Autodesk Inventor part; units mm, degrees
ref_plane "YZ Plane" through (0, 0, 0) normal (1, 0, 0) x (0, 1, 0)
ref_plane "XZ Plane" through (0, 0, 0) normal (0, 1, 0) x (-1, 0, 0)
ref_plane "XY Plane" through (0, 0, 0) normal (0, 0, 1) x (1, 0, 0)
sketch "Sketch1" plane through (0, 0, 0) normal (0, 1, 0) x (-1, 0, 0)
  line L0 (19.304, 65.405) -> (-19.304, 65.405)
  line L1 (-19.304, 65.405) -> (-19.304, -65.405)
  line L2 (-19.304, -65.405) -> (19.304, -65.405)
  line L3 (19.304, -65.405) -> (19.304, 65.405)
  line L4 (19.304, 65.405) -> (-19.304, -65.405) construction
  line L5 (-19.304, 65.405) -> (19.304, -65.405) construction
  line L6 (21.209, 67.31) -> (-21.209, 67.31)
  line L7 (-21.209, 67.31) -> (-21.209, -67.31)
  line L8 (-21.209, -67.31) -> (21.209, -67.31)
  line L9 (21.209, -67.31) -> (21.209, 67.31)
  point P0 (0, 0)
  dimension "d0" = 38.608
  dimension "d1" = 130.81
  dimension "d2" = 1.905
extrude "Extrusion1" add sketch "Sketch1" along normal blind 20.32
extrude "Extrusion2" add sketch "Sketch1" along normal blind 1.905 contours L3 L2 L1 L0
sketch "Sketch2" plane through (21.209, 0, 67.31) normal (1, 0, 0) x (0, 0, -1)
  line L0 (12.7, 20.32) -> (121.92, 20.32)
  line L1 (121.92, 20.32) -> (121.92, 7.62)
  line L2 (121.92, 7.62) -> (12.7, 7.62)
  line L3 (12.7, 7.62) -> (12.7, 20.32)
  line L4 (0, 0) -> (0, 20.32)
  line L5 (134.62, 0) -> (134.62, 20.32)
  line L6 (0, 20.32) -> (134.62, 20.32)
  line L7 (0, 0) -> (134.62, 0)
  point P0 (67.31, 0)
  dimension "d7" = 12.7
  dimension "d8" = 12.7
  dimension "d9" = 7.62
extrude "Extrusion3" cut sketch "Sketch2" against normal blind 1.905 contours L0 L1 L2 L3
sketch "Sketch3" plane through (-21.209, 0, -67.31) normal (-1, 0, 0) x (0, 0, 1)
  line L0 (12.7, 20.32) -> (121.92, 20.32)
  line L1 (121.92, 20.32) -> (121.92, 5.08)
  line L2 (121.92, 5.08) -> (12.7, 5.08)
  line L3 (12.7, 5.08) -> (12.7, 20.32)
  line L4 (0, 20.32) -> (134.62, 20.32)
  line L5 (0, 0) -> (0, 20.32)
  line L6 (134.62, 0) -> (134.62, 20.32)
  line L7 (0, 0) -> (134.62, 0)
  point P0 (67.31, 0)
  dimension "d12" = 12.7
  dimension "d13" = 12.7
  dimension "d14" = 5.08
extrude "Extrusion4" cut sketch "Sketch3" against normal blind 1.905 contours L0 L1 L2 L3
sketch "Sketch4" plane through (0, 20.32, 0) normal (0, 1, 0) x (1, 0, 0)
  line L0 (21.209, 67.31) -> (-21.209, 67.31)
  line L1 (-19.304, 65.405) -> (19.304, 65.405)
  line L2 (14.224, 67.31) -> (11.176, 67.31)
  line L3 (11.176, 67.31) -> (11.176, 65.405)
  line L4 (11.176, 65.405) -> (14.224, 65.405)
  line L5 (14.224, 65.405) -> (14.224, 67.31)
  line L6 (19.304, 65.405) -> (19.304, 54.61)
  line L7 (-19.304, 54.61) -> (-19.304, 65.405)
  point P0 (0, 0)
  dimension "d17" = 5.08
  dimension "d18" = 30.48
extrude "Extrusion5" cut sketch "Sketch4" against normal up to surface (18.415 mm away)
sketch "Sketch5" plane through (21.209, 0, -67.31) normal (0, 0, -1) x (-1, 0, 0)
  line L0 (0, 0) -> (42.418, 0)
  line L1 (0, 0) -> (42.418, 0)
  line L2 (42.418, 0) -> (42.418, 1.905)
  line L3 (42.418, 1.905) -> (0, 1.905)
  line L4 (0, 1.905) -> (0, 0)
  line L5 (10.033, 1.905) -> (6.985, 1.905)
  line L6 (42.418, 0) -> (42.418, 20.32)
  point P0 (21.209, 0)
extrude "Extrusion6" add sketch "Sketch5" along normal blind 24.13
sketch "Sketch6" plane through (0, 1.905, 0) normal (0, 1, 0) x (1, 0, 0)
  line L0 (-19.558, 76.835) -> (4.064, 76.835)
  line L1 (4.064, 76.835) -> (4.064, 89.789)
  line L2 (4.064, 89.789) -> (-19.558, 89.789)
  line L3 (-19.558, 89.789) -> (-19.558, 76.835)
  line L4 (19.304, 65.405) -> (19.304, 54.61)
  line L5 (11.176, 67.31) -> (-21.209, 67.31)
  line L6 (-21.209, 75.184) -> (5.715, 75.184)
  line L7 (5.715, 75.184) -> (5.715, 91.44)
  line L8 (5.715, 91.44) -> (-21.209, 91.44)
  line L9 (-21.209, 91.44) -> (-21.209, 75.184)
  line L10 (-21.209, 91.44) -> (21.209, 91.44)
  line L11 (-21.209, 67.31) -> (-21.209, 91.44)
  line L12 (-19.304, 65.405) -> (11.176, 65.405)
  point P0 (0, 0)
  dimension "d24" = 12.954
  dimension "d26" = 23.622
  dimension "d32" = 11.43
extrude "Extrusion7" add sketch "Sketch6" along normal blind 33.02
sketch "Sketch8" plane through (4.064, 1.905, -89.789) normal (-1, 0, 0) x (0, 0, 1)
  circle A0 centre (6.477, 20.32) radius 6.477
  line L0 (0, 0) -> (0, 33.02)
  line L1 (12.954, 0) -> (12.954, 33.02)
  line L2 (0, 0) -> (12.954, 0)
  line L3 (12.954, 20.32) -> (12.954, 33.02)
  line L4 (0, 33.02) -> (0, 20.32)
  line L5 (12.954, 33.02) -> (0, 33.02)
  line L6 (12.954, 20.32) -> (12.954, 33.02)
  line L7 (0, 33.02) -> (0, 20.32)
  point P0 (89.789, -1.905)
  dimension "d29" = 20.32
extrude "Extrusion8" cut sketch "Sketch8" against normal blind 33.02 contours A0 | A0 L0 L5 L1
sketch "Sketch10" plane through (4.064, 1.905, -89.789) normal (-1, 0, 0) x (0, 0, 1)
  line L0 (-1.651, 0) -> (14.605, 0)
  line L1 (-1.651, 0) -> (-1.651, 33.02)
  line L2 (14.605, 0) -> (-1.651, 0)
  line L3 (-1.651, 0) -> (-1.651, 13.208)
  line L4 (-1.651, 13.208) -> (14.605, 13.208)
  line L5 (14.605, 13.208) -> (14.605, 0)
  arc A0 (0, 20.32) -> (12.954, 20.32) centre (6.477, 20.32) ccw
  point P0 (89.789, -1.905)
  point P1 (6.477, 13.843)
  point P2 (6.477, 13.208)
  dimension "d37" = 0.635
extrude "Extrusion10" add sketch "Sketch10" along normal blind 3.048
sketch "Sketch9" plane through (5.715, 1.905, -75.184) normal (1, 0, 0) x (0, 0, -1)
  arc A0 (1.651, 20.32) -> (14.605, 20.32) centre (8.128, 20.32) ccw
  circle A1 centre (8.372, 11.303) radius 1.524
  point P0 (-75.184, -1.905)
  point P1 (8.128, 13.843)
  dimension "d33" = 2.54
  dimension "d34" = 3.048
extrude "Extrusion9" cut sketch "Sketch9" against normal up to surface (25.273 mm away)
sketch "Sketch11" plane through (21.209, 0, 67.31) normal (1, 0, 0) x (0, 0, -1)
  line L0 (134.62, 1.905) -> (158.75, 1.905)
  line L1 (0, 0) -> (158.75, 0)
  line L2 (158.75, 0) -> (158.75, 1.905)
  line L3 (158.75, 1.905) -> (0, 1.905)
  line L4 (0, 1.905) -> (0, 0)
  point P0 (67.31, 0)
extrude "Extrusion11" add sketch "Sketch11" along normal blind 76.2
sketch "Sketch12" plane through (0, 1.905, 0) normal (0, 1, 0) x (1, 0, 0)
  circle A0 centre (91.059, -43.815) radius 3.81
  line L0 (21.209, 54.61) -> (21.209, -54.61)
  line L1 (19.304, -65.405) -> (-19.304, -65.405)
  line L2 (21.209, -51.435) -> (97.409, -51.435)
  line L3 (97.409, 91.44) -> (97.409, -67.31)
  line L4 (97.409, -67.31) -> (21.209, -67.31)
  line L5 (21.209, -67.31) -> (21.209, -51.435)
  line L6 (97.409, -36.195) -> (21.209, -36.195)
  line L7 (-21.209, 91.44) -> (97.409, 91.44)
  line L8 (21.209, 91.44) -> (97.409, 91.44)
  line L9 (97.409, 91.44) -> (97.409, -36.195)
  line L10 (21.209, -36.195) -> (97.409, -36.195)
  line L11 (97.409, -36.195) -> (97.409, 91.44)
  line L12 (97.409, 91.44) -> (21.209, 91.44)
  line L13 (21.209, 91.44) -> (21.209, -36.195)
  line L14 (5.715, 91.44) -> (97.409, 91.44)
  line L15 (97.409, 91.44) -> (97.409, 67.31)
  line L16 (5.715, 67.31) -> (5.715, 91.44)
  line L17 (5.715, 89.789) -> (5.715, 91.44)
  line L18 (21.209, 67.31) -> (14.224, 67.31)
  circle A1 centre (65.659, -34.29) radius 3.81
  circle A2 centre (91.059, -24.765) radius 3.81
  circle A3 centre (91.059, -5.715) radius 3.81
  circle A4 centre (91.059, 13.335) radius 3.81
  circle A5 centre (91.059, 32.385) radius 3.81
  circle A6 centre (65.659, -15.24) radius 3.81
  circle A7 centre (65.659, 3.81) radius 3.81
  circle A8 centre (65.659, 22.86) radius 3.81
  circle A9 centre (65.659, 41.91) radius 3.81
  line L19 (21.209, 91.44) -> (97.409, 91.44)
  line L20 (97.409, 91.44) -> (97.409, 49.53)
  line L21 (97.409, 49.53) -> (21.209, 49.53)
  line L22 (21.209, 49.53) -> (21.209, 91.44)
  line L23 (5.715, 67.31) -> (21.209, 67.31)
  line L24 (21.209, 67.31) -> (21.209, 91.44)
  line L25 (21.209, 91.44) -> (5.715, 91.44)
  line L26 (5.715, 91.44) -> (5.715, 67.31)
  point P0 (0, 0)
  point P1 (97.409, -36.195)
  point P2 (21.209, -54.61)
  point P3 (5.715, 90.6145)
  point P4 (21.209, 49.53)
  dimension "d42" = 7.62
  dimension "d44" = 21.59
  dimension "d45" = 7.62
  dimension "d46" = 7.62
  dimension "d59" = 7.62
  dimension "d76" = 69.85
  dimension "d79" = 19.05
  dimension "d84" = 9.525
  dimension "d87" = 19.05
  dimension "d92" = 25.4
  dimension "d93" = 7.62
extrude "Extrusion12" cut sketch "Sketch12" against normal blind 57.15 contours A0 | L13 L7 L3 L21 L0 | L18 L23 L16 L7 L13 | L2 L3 L4 L5 L0 | A1 L6 | L6 A1 | A2 | A3 | A4 | A5 | A6 | A7 | A8 | A9
sketch "Sketch13" plane through (0, 1.905, 0) normal (0, 1, 0) x (1, 0, 0)
  line L0 (11.176, 67.31) -> (-21.209, 67.31)
  line L1 (-21.209, 75.184) -> (5.715, 75.184)
  line L2 (-13.589, 67.31) -> (-1.905, 67.31)
  line L3 (-1.905, 67.31) -> (-1.905, 75.184)
  line L4 (-1.905, 75.184) -> (-13.589, 75.184)
  line L5 (-13.589, 75.184) -> (-13.589, 67.31)
  line L6 (-21.209, 67.31) -> (-21.209, 75.184)
  line L7 (5.715, 91.44) -> (5.715, 75.184)
  point P0 (0, 0)
  point P1 (-21.209, 71.247)
  point P2 (-13.589, 71.247)
  point P3 (5.715, 67.31)
  point P4 (-1.905, 67.31)
  dimension "d49" = 7.62
  dimension "d50" = 7.62
extrude "Extrusion13" add sketch "Sketch13" along normal blind 12.7
properties part number "HarmonicaFrame"
Read the model definition and answer for the solid it produces. Units are mm, in the model's axes. A direction names the side the tool comes from. Round coordinates to 2 decimals unless told otherwise and drop trailing zeros. Write each loop counter-clockwise with the first axis right and the second up, starting at its lowest first coordinate (ties: lowest second). Pieces come first, ordered by that corner, then holes. Notation, with made-up numbers: M -11.75,-17.5 L 18.25,-17.5 A18 cw 18.25,14.5 Z; hole C 10,77 d10. An arc over 180 degrees is marked long. One line per item, written item: value.
Q1. For a pull along X with two mould halves and no side action, classify faces 1 (the cylindrical face through (3.398, 13.275, -82.033)), 2 (the cylindrical face through (94.693, 0.966, 42.671)) as +X half, -X half, draft (parallel to the pull), parting line (faces both ways), or undercut.
Data:
face 1: draft
face 2: undercut
Q2. Flat-ended cylindrical pins translate along their axes: pin 1 Ø0.6 at (x, y) = (53.5, 1) entering from +Z (3 decimals); pin 2 Ø1 at (x, z) = (41, -40.5) entering from +Y (3 decimals); pin 3 Ø2 at (y, z) = (7.5, -48.5) entering from +X; pin 4 Ø6 at (x, z) = (1.5, -38.5) entering from -Y. Find the tip coordinate at first contact, or state that the pin passes through.
Data:
pin 1: z = 51.435
pin 2: y = 1.905
pin 3: x = 21.21
pin 4: y = 0
Q3. Find section D-D on z = -72.5. Write down the section's boundary in (x, y) (3 decimals), plus the area to 3 significant figures.
Data:
outline: M -21.209,0 L 5.715,0 L 5.715,1.905 L -1.905,1.905 L -1.905,14.605 L -21.209,14.605 Z
area: 296 mm2
Q4. Find section B-B on x = 65. Write down the section's boundary in (y, z) (3 decimals), plus the area to 3 significant figures.
Data:
outline: M 0,-49.53 L 1.905,-49.53 L 1.905,-45.663 L 0,-45.663 Z; M 0,-38.157 L 1.905,-38.157 L 1.905,-26.613 L 0,-26.613 Z; M 0,-19.107 L 1.905,-19.107 L 1.905,-7.563 L 0,-7.563 Z; M 0,-0.057 L 1.905,-0.057 L 1.905,11.487 L 0,11.487 Z; M 0,18.993 L 1.905,18.993 L 1.905,30.537 L 0,30.537 Z; M 0,38.043 L 1.905,38.043 L 1.905,51.435 L 0,51.435 Z
area: 121 mm2
Q5. Straight lines are drawn through the part: line 1 (Z direction, x = -8, y = 6) (3 decimals); line 2 (Z direction, x = -10, y = 15.5) (3 decimals); line 3 (Z direction, x = 4, y = 30) (3 decimals). For each, find the intervals that lie inside material, in ascending order. Write a range as [from, to].
Data:
line 1: [-91.44, -89.789], [-76.835, -65.405], [65.405, 67.31]
line 2: [-91.44, -89.789], [-76.835, -75.184], [-67.31, -65.405], [65.405, 67.31]
line 3: [-91.44, -89.789], [-76.835, -75.184]
Q6. Which of the six approach directions +Z, -Z, +X, -X, +Y, -Y give full straight-line access (tool end or side, diameter ignored) to faces 3 (the flat face through (5, 12, -67.31)), 4 (the flat face through (1.016, 9, -83)), 5 (the flat face through (-12, 14.605, -71)), 6 (the flat face through (-9, 20.32, -66))?
Data:
face 3: +X, +Y
face 4: +Y
face 5: +X, -X, +Y
face 6: +Z, +X, -X, +Y
Q7. Find section A-A on z = -41.91. Write down the section's boundary in (x, y) (3 decimals), plus the area to 3 significant figures.
Data:
outline: M -21.209,0 L 61.849,0 L 61.849,1.905 L 21.209,1.905 L 21.209,7.62 L 19.304,7.62 L 19.304,1.905 L -19.304,1.905 L -19.304,5.08 L -21.209,5.08 Z; M 69.469,0 L 97.409,0 L 97.409,1.905 L 69.469,1.905 Z
area: 228 mm2
Q8. Find section C-C on y = 27. Write down the section's boundary in (x, z) (3 decimals).
Data:
outline: M -21.209,-91.44 L 5.715,-91.44 L 5.715,-89.789 L -19.558,-89.789 L -19.558,-76.835 L 5.715,-76.835 L 5.715,-75.184 L -21.209,-75.184 Z
